Autodesk Inventor part; units mm, degrees
ref_plane "Plan de construction3" through (-65, 30, 0) normal (0, 1, 0) x (1, 0, 0)
ref_plane "Plan de construction4" through (11.8427, 40, 20) normal (0, 0, 1) x (1, 0, 0)
ref_plane "YZ Plane" through (0, 0, 0) normal (1, 0, 0) x (0, 1, 0)
sketch "Esquisse8" plane through (0, 0, 0) normal (0, 0, 1) x (1, 0, 0)
  line L0 (65, -20) -> (65, 40)
  line L1 (65, 40) -> (-65, 40)
  line L2 (-65, 40) -> (-65, -20)
  line L3 (-45, 20) -> (45, 20)
  line L4 (-45, 20) -> (-45, -20)
  line L5 (45, 20) -> (45, -20)
  line L6 (65, -20) -> (45, -20)
  line L7 (-45, -20) -> (-65, -20)
  point P0 (0, 0)
  dimension "d45" = 20
  dimension "d46" = 90
  dimension "d47" = 45
  dimension "d71" = 20
  dimension "d72" = 20
extrude "Extrusion7" add sketch "Esquisse8" along normal blind 60
sketch "Esquisse10" plane through (0, 0, 0) normal (0, 0, -1) x (-1, 0, 0)
  line L0 (45, 20) -> (-45, 20)
  line L1 (-55, 30) -> (-55, 10)
  line L2 (55, 10) -> (55, 30)
  line L3 (-55, 10) -> (-55, -10)
  line L4 (55, 10) -> (55, -10)
  dimension "d75" = 20
  dimension "d80" = 20
  dimension "d89" = 20
  dimension "d90" = 20
hole "Perçage2" at (55, 10, 0) at (-55, 10, 0) at (-55, 30, 0) at (55, 30, 0) at (-55, -10, 0) at (55, -10, 0) direction (0, 0, 1) diameter 6 end through all counterbore diameter 10 counterbore depth 4
sketch "Esquisse13" plane through (-65, 40, 0) normal (0, 1, 0) x (1, 0, 0)
  line L0 (65, 0) -> (65, -20)
  circle A0 centre (65, -20) radius 4
  dimension "d81" = 20
  dimension "d82" = 8
extrude "Extrusion9" cut sketch "Esquisse13" against normal up to surface (20 mm away)
sketch "Esquisse14" plane through (-65, 40, 0) normal (0, 1, 0) x (1, 0, 0)
  circle A0 centre (65, -20) radius 4
  line L0 (0, 0) -> (130, 0)
  line L1 (0, 0) -> (0, -60)
  line L2 (130, -60) -> (0, -60)
  line L3 (130, 0) -> (130, -60)
  circle A1 centre (65, -20) radius 9.5
  point P0 (65, 0)
  dimension "d85" = 19
extrude "Extrusion10" cut sketch "Esquisse14" against normal blind 6 contours A1
ref_plane "Plan de construction3" through (-65, 30, 0) normal (0, 1, 0) x (1, 0, 0)
mirror "Symétrie5" about plane through (-65, 30, 0) normal (0, 1, 0) of "Extrusion10"
sketch "Esquisse15" plane through (-65, 40, 0) normal (0, 1, 0) x (1, 0, 0)
  circle A0 centre (65, -20) radius 9.5
  circle A1 centre (65, -20) radius 15.5
  line L0 (130, -60) -> (0, -60)
  line L1 (0, 0) -> (130, 0)
  line L2 (130, 0) -> (130, -10)
  line L3 (130, -30) -> (130, -60)
  line L4 (0, 0) -> (0, -10)
  line L5 (0, -30) -> (0, -60)
  line L6 (130, -30) -> (76.8427, -30)
  line L7 (53.1573, -30) -> (0, -30)
  line L8 (0, -10) -> (53.1573, -10)
  line L9 (76.8427, -10) -> (130, -10)
  point P0 (65, 0)
  dimension "d91" = 6
extrude "Extrusion11" cut sketch "Esquisse15" against normal through all contours A1 L8 L4 L1 L2 L9 | L6 L3 L0 L5 L7 A1
sketch "Esquisse16" plane through (65, 40, 10) normal (0, 0, -1) x (-1, 0, 0)
  circle A0 centre (10, -50) radius 3
  circle A1 centre (10, -30) radius 3
  circle A2 centre (10, -10) radius 3
  circle A3 centre (120, -10) radius 3
  circle A4 centre (120, -30) radius 3
  circle A5 centre (120, -50) radius 3
  circle A6 centre (10, -50) radius 5
  circle A7 centre (10, -30) radius 5
  circle A8 centre (10, -10) radius 5
  circle A9 centre (120, -10) radius 5
  circle A10 centre (120, -30) radius 5
  circle A11 centre (120, -50) radius 5
  point P0 (65, -40)
  dimension "d96" = 10
  dimension "d97" = 10
extrude "Extrusion12" cut sketch "Esquisse16" against normal blind 4 contours A0 | A1 | A2 | A3 | A4 | A5 | A6 | A7 | A8 | A9 | A10 | A11
ref_plane "Plan de construction4" through (11.8427, 40, 20) normal (0, 0, 1) x (1, 0, 0)
mirror "Symétrie6" about plane through (11.8427, 40, 20) normal (0, 0, 1) of "Extrusion12"
chamfer "Chanfrein1" distance 2 angle 45 4 edges at (11.8427, 30, 10) (11.8427, 30, 30) (-11.8427, 30, 30) (-11.8427, 30, 10)
chamfer "Chanfrein2" distance 6 angle 45 4 edges at (65, -20, 20) (45, -20, 20) (-45, -20, 20) (-65, -20, 20)
properties part number "Block1"
The model under review builds one solid part; all positions refer to its coordinate system, in mm. A direction names the side the tool comes from. Give positions to 0.01 mm unless a question says otherwise; leave off trailing zeros. Loops run counter-clockwise (first coordinate to the right, second up) from the corner with the lowest first, then second, coordinate; pieces in that order, holes last. Notation, with made-up numbers: (39.5, -13) -> (98.5, -13) arc R24 ccw to (98.5, 2) -> close; hole circle Ø1 at (61.25, 47.25). An arc over 180 degrees is marked (long way). Put each result on its own line as item: value. Start each with the question number.
1. For faces 5 (the face through (45, 3, 20)), 6 (the face through (9.061, 37.042, 17.146)), 7 (the face through (-51.7, -9.9, 26)), 8 (the face through (-58.3, 10.1, 14)), list the 3-axis set-ups (+Z, -Z, +X, -X, +Y, -Y) from which the entire face can be reached by the end or side of a thin tool; tool diameter is ignored.
2. We need section C-C on x = 0. State the section outline as (y, z) points, then the cut area to 3 significant figures.
3. We need section A-A on z = 20. State how many separate pieces and enclosed holes the cut face has, then the cut area to 3 significant figures.
4. Mouldability with a two-part tool opening along Z and no side actions: class faces 1 (the face through (-12.2, 30.1, 30.7)), 2 (the face through (55, -20, 20)), 3 (the face through (-4, 26, 22)), 4 (the face through (51.7, -9.9, 14)) as released by +Z, released by -Z, zero draft, split by the parting line, or undercut.
5. We need section B-B on y = -2. State the section outline as (x, z) points.
6. Clearance check with flat-ended pins moving along their axes: P1, Ø9, axis at x = 55, y = -10, coming from the +Z side; P2, Ø11.5, axis at x = -55, y = 10, coming from the +Z side; P3, Ø1.5, axis at x = 18.5, z = 27, coming from the -Y side. State where each tip first meets the part, or that it passes through.
7. Wall thickness on probe 1 along Y at (x, z) = (-55, 22.5); probe 2 along X at (y, z) = (-10, 23.25); probe 3 along Y at (x, z) = (-55, 28.65): over which ranges is each line inside the solid? List them lowest first.
Determined:
1. face 5: +Z, -Z, -Y
1. face 6: +Y
1. face 7: +Z
1. face 8: -Z
2. outline: (20, 4.5) -> (40, 4.5) -> (40, 10.5) -> (34, 10.5) -> (34, 16) -> (26, 16) -> (26, 10.5) -> (20, 10.5) -> close; (20, 29.5) -> (26, 29.5) -> (26, 24) -> (34, 24) -> (34, 29.5) -> (40, 29.5) -> (40, 35.5) -> (20, 35.5) -> close
2. area: 328 mm^2
3. separate pieces: 2
3. enclosed holes: 6
3. area: 3,670 mm^2
4. face 1: released by +Z
4. face 2: zero draft
4. face 3: undercut
4. face 4: released by -Z
5. outline: (-65, 10) -> (-45, 10) -> (-45, 30) -> (-65, 30) -> close; (45, 10) -> (65, 10) -> (65, 30) -> (45, 30) -> close
6. P1: z = 26
6. P2: z = 30
6. P3: y = 20
7. probe 1: -20 to -13, -7 to 7, 13 to 27, 33 to 40
7. probe 2: -65 to -58, -52 to -45, 45 to 52, 58 to 65
7. probe 3: -20 to -15, -5 to 5, 15 to 25, 35 to 40
